Part model, mm, in its own coordinate system. Give positions to 0.01 mm unless a question says otherwise; leave off trailing zeros. Loops run counter-clockwise (first coordinate to the right, second up) from the corner with the lowest first, then second, coordinate; pieces in that order, holes last. Notation, with made-up numbers: (79, 47.25) -> (109, 47.25) arc R4 cw to (109, 51.25) -> close; hole circle Ø4 at (12.5, 81.5). An arc over 180 degrees is marked (long way). Write item = value, one per line.
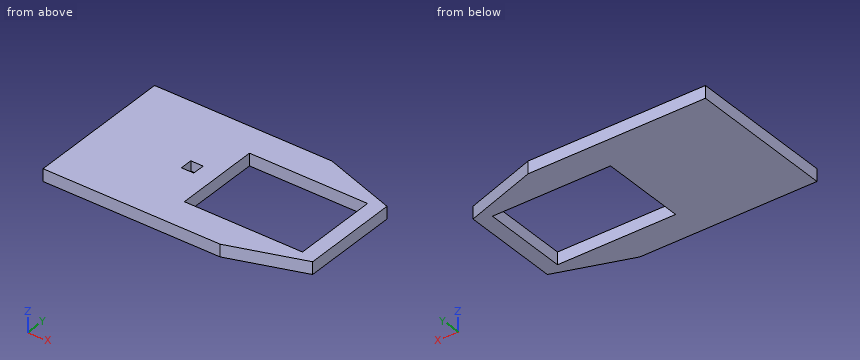
from build123d import *

# Parameters (mm, degrees)
F0_W     = 102
F0_H     = 60
F0_W_2   = 48
F0_H_2   = 35
F1_DEPTH = 5
F3_DEPTH = 4
F4_SIZE2 = 30
F4_SIZE  = 10


with BuildPart() as f1:
    # F0 (on Top) → F1 (new body)
    with BuildSketch(Plane.XY):
        with Locations((-63.9077364467, 31.1956779382)):
            Rectangle(F0_W, F0_H)
        with Locations((-42.9077364467, 31.1956779382)):
            Rectangle(F0_W_2, F0_H_2, mode=Mode.SUBTRACT)
    extrude(amount=F1_DEPTH)

    # F2 (on face) → F3 (cut)
    with BuildSketch(Plane.XY.offset(5)):
        Polygon((-74.3977364467, 33.7056779382), (-79.4177364467, 33.7056779382), (-79.4177364467, 28.6856779382), (-74.3977364467, 28.6856779382), (-74.3977364467, 31.1956779382), align=None)
    extrude(amount=-F3_DEPTH, mode=Mode.SUBTRACT)

    # F4
    f4_edges = [f1.edges().sort_by_distance(p)[0] for p in [
        (-12.907736, 1.195678, 2.5),
        (-12.907736, 61.195678, 2.5),
    ]]
    f4_side = f1.faces().sort_by_distance((-12.907736, 31.195678, 2.5))[0]
    chamfer(f4_edges, length=F4_SIZE, length2=F4_SIZE2, reference=f4_side)


solid = f1.part
1) Slice it at D-D, the plane y = 54. List the corners of the cut face in (x, z).
Resolved:
outline = (-114.91, 0) -> (-21.32, 0) -> (-21.32, 5) -> (-114.91, 5) -> close
2) Slice it at C-C, the plane x = -20. List the corners of the cut face in (y, z), and give its area (3 significant figures).
Resolved:
outline = (8.83, 0) -> (13.7, 0) -> (13.7, 5) -> (8.83, 5) -> close; (48.7, 0) -> (53.56, 0) -> (53.56, 5) -> (48.7, 5) -> close
area = 48.6 mm²
3) Slice it at A-A, the plane y = 17. List the corners of the cut face in (x, z), and give its area (3 significant figures).
Resolved:
outline = (-114.91, 0) -> (-66.91, 0) -> (-66.91, 5) -> (-114.91, 5) -> close; (-18.91, 0) -> (-12.91, 0) -> (-12.91, 5) -> (-18.91, 5) -> close
area = 270 mm²
4) Drill centre lines: line 1 along X through (y, z) = (32.5, 4.4); line 2 along Y through (x, z) = (-44, 4.2); line 3 along X through (y, z) = (36, 4.65). Where is each one in solid material? Low to high. Write a range as [from, to].
Resolved:
line_1 = [-114.91, -79.42], [-74.4, -66.91], [-18.91, -12.91]
line_2 = [1.2, 13.7], [48.7, 61.2]
line_3 = [-114.91, -66.91], [-18.91, -12.91]
5) Drop flat-ended pins along their axis: P1, Ø1.5, axis at x = -42, z = 4.5, coming from the -Y side; P2, Ø2.5, axis at x = -77, y = 30, coming from the +Z side. Give the stop position or say it passes through.
Resolved:
P1 = 1.25
P2 = 1
6) Slice it at B-B, the plane z = 2.55. List the corners of the cut face in (x, y), and give its area (3 significant figures).
Resolved:
outline = (-114.91, 1.2) -> (-42.91, 1.2) -> (-12.91, 11.2) -> (-12.91, 51.2) -> (-42.91, 61.2) -> (-114.91, 61.2) -> close; hole (-79.42, 28.69) -> (-74.4, 28.69) -> (-74.4, 33.71) -> (-79.42, 33.71) -> close; hole (-66.91, 13.7) -> (-18.91, 13.7) -> (-18.91, 48.7) -> (-66.91, 48.7) -> close
area = 4,110 mm²
